Check sheet for the modelled part. Datum: model origin and axes. Units: mm. Face numbers are marked on the shaded views. Round coordinates to 2 decimals unless told otherwise and drop trailing zeros. Loops run counter-clockwise (first coordinate to the right, second up) from the corner with the lowest first, then second, coordinate; pieces in that order, holes last. Notation, with made-up numbers: (-37, -4.75) - (-29, -4.75) arc R12 ccw to (-29, 13.25) - close; hole circle Ø6 at (-22, -18). An arc over 180 degrees is marked (long way). Answer in a Markdown table with one row per item. Add a question column.
(1) Cross-section at A-A on x = 0. Enter the section's corners in (y, z).
(2) Gauge pin test, flat ends, axial feed: pin 1 (12 mm diameter, centred on x = -10.5, y = 95, fed in from -Z); pin 2 (4 mm diameter, centred on y = 221.5, z = -7.5, fed in from -X); pin 3 (3 mm diameter, centred on x = -4.5, y = 111, fed in from -Z). Record the tip position at first contact, or that the pin passes through.
(3) Thickness scan on line 1 along X through (y, z) = (125, 0); line 2 along Z through (x, y) = (-6.5, 113.5); line 3 along X through (y, z) = (262.5, 4). Record the ranges inside material, lowest first.
(4) Cross-section at C-C on y = 29.5. Enter the section's corners in (x, z).
(5) Mould release check, pull along Z, two halves, no side actions. Record for the marked faces 1 and 2: +Z half, -Z half, draft (parallel to the pull), parting line (faces both ways), or undercut.
(6) Cross-section at B-B on z = 0. Enter the section's corners in (x, y), then the cut area to 3 significant figures.
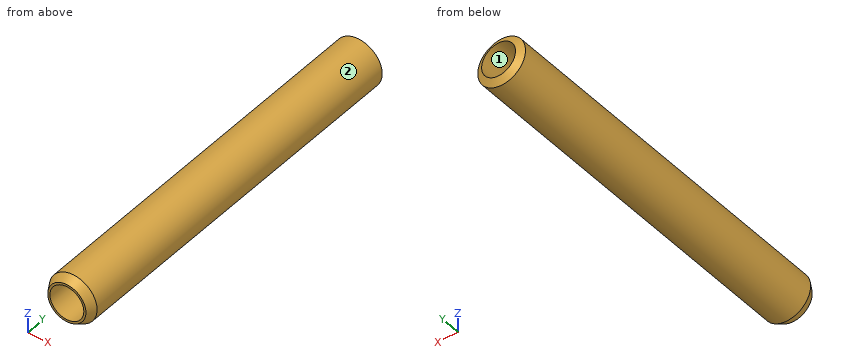
from build123d import *

# Parameters (mm, degrees)
SKETCH1_R           = 17.5
BOSS_EXTRUDE1_DEPTH = 279.982262
SKETCH2_R           = 12.415069034
CUT_EXTRUDE1_DEPTH  = 282.073952964
CHAMFER1_SIZE       = 3.490287
CHAMFER1_SIZE_2     = 6.045354


with BuildPart() as part:
    # Sketch1 → Boss-Extrude1 (new body)
    with BuildSketch(Plane(origin=(0, 0, 0), x_dir=(1, 0, 0), z_dir=(0, 1, 0))):
        with Locations(Location((0, 0, 0), (0, 0, 270))):
            Circle(SKETCH1_R)
    extrude(amount=BOSS_EXTRUDE1_DEPTH)

    # Sketch2 → Cut-Extrude1 (cut, through all)
    with BuildSketch(Plane(origin=(0, 0, 0), x_dir=(1, 0, 0), z_dir=(0, 1, 0))):
        with Locations(Location((0, 0, 0), (0, 0, 270))):
            Circle(SKETCH2_R)
    extrude(amount=CUT_EXTRUDE1_DEPTH, mode=Mode.SUBTRACT)

    # Chamfer1
    # the kernel refuses this chamfer: 6.045354, 3.490287 mm, written as the material it takes off along each edge
    with BuildSketch(Plane(origin=(0, 279.982262, 0), x_dir=(0, 0, 1), z_dir=(-1, 0, 0))) as chamfer1_piece_1:
        Polygon((17.5, -CHAMFER1_SIZE), (17.5 - CHAMFER1_SIZE_2, 0), (17.5, 0), align=None)
    revolve(axis=Axis((0, 279.982262, 0), (0, 1, 0)), mode=Mode.SUBTRACT)
    with BuildSketch(Plane(origin=(0, 0, 0), x_dir=(0, 0, 1), z_dir=(-1, 0, 0))) as chamfer1_piece_2:
        Polygon((17.5, CHAMFER1_SIZE_2), (17.5 - CHAMFER1_SIZE, 0), (17.5, 0), align=None)
    revolve(axis=Axis((0, 0, 0), (0, 1, 0)), mode=Mode.SUBTRACT)


solid = part.part
Answers:
| question | item | result |
|---|---|---|
| 1 | outline | (0, -14.01) - (6.05, -17.5) - (276.49, -17.5) - (279.43, -12.42) - (0, -12.42) - close; (0, 12.42) - (279.43, 12.42) - (276.49, 17.5) - (6.05, 17.5) - (0, 14.01) - close |
| 2 | pin 1 | stops at z = -16.91 |
| 2 | pin 2 | stops at x = -16.61 |
| 2 | pin 3 | stops at z = -17.24 |
| 3 | line 1 | x = -17.5 to -12.42, 12.42 to 17.5 |
| 3 | line 2 | z = -16.25 to -10.58, 10.58 to 16.25 |
| 3 | line 3 | x = -17.04 to -11.75, 11.75 to 17.04 |
| 4 | outline | circle Ø35 at (0, 0); hole circle Ø24.83 at (0, 0) |
| 5 | face 1 | undercut |
| 5 | face 2 | parting line |
| 6 | outline | (-17.5, 6.05) - (-14.01, 0) - (-12.42, 0) - (-12.42, 279.43) - (-17.5, 276.49) - close; (12.42, 0) - (14.01, 0) - (17.5, 6.05) - (17.5, 276.49) - (12.42, 279.43) - close |
| 6 | area | 2,810 mm^2 |
